Part model, mm, in its own coordinate system. Give positions to 0.01 mm unless a question says otherwise; leave off trailing zeros. Loops run counter-clockwise (first coordinate to the right, second up) from the corner with the lowest first, then second, coordinate; pieces in that order, holes last. Notation, with made-up numbers: M 23.5,77 L 28.5,77 A24 ccw 28.5,91 Z; hole C 54,2.25 d2. An arc over 180 degrees is marked long. Answer in a Markdown table with one row per item.
Autodesk Inventor part; units mm, degrees
ref_plane "YZ Plane" through (0, 0, 0) normal (1, 0, 0) x (0, 1, 0)
ref_plane "XZ Plane" through (0, 0, 0) normal (0, 1, 0) x (-1, 0, 0)
ref_plane "XY Plane" through (0, 0, 0) normal (0, 0, 1) x (1, 0, 0)
sketch "Sketch1" plane through (0, 0, 0) normal (0, 1, 0) x (-1, 0, 0)
  line L0 (38.1, 76.2) -> (-38.1, 76.2)
  line L1 (-38.1, 76.2) -> (-38.1, -76.2)
  line L2 (-38.1, -76.2) -> (38.1, -76.2)
  line L3 (38.1, -76.2) -> (38.1, 76.2)
  line L4 (38.1, 76.2) -> (-38.1, -76.2) construction
  line L5 (-38.1, 76.2) -> (38.1, -76.2) construction
  point P0 (0, 0)
  dimension "d0" = 76.2
  dimension "d1" = 152.4
extrude "Extrusion1" add sketch "Sketch1" along normal blind 6.35
sketch "Sketch2" plane through (0, 6.35, 0) normal (0, 1, 0) x (1, 0, 0)
  line L0 (38.1, 76.2) -> (-38.1, 76.2)
  line L1 (-38.1, 76.2) -> (-38.1, -76.2)
  line L2 (38.1, -76.2) -> (38.1, 76.2)
  line L3 (-38.1, -76.2) -> (38.1, -76.2)
  point P0 (0, 0)
  point P1 (-25.4, 63.5)
  point P2 (25.4, 63.5)
  point P3 (25.4, -63.5)
  point P4 (-25.4, -63.5)
  dimension "d11" = 12.7
  dimension "d12" = 12.7
  dimension "d13" = 12.7
  dimension "d14" = 12.7
  dimension "d15" = 12.7
  dimension "d16" = 12.7
  dimension "d17" = 12.7
  dimension "d18" = 12.7
hole "Hole1" at (-25.4, 6.35, -63.5) at (25.4, 6.35, -63.5) at (25.4, 6.35, 63.5) at (-25.4, 6.35, 63.5) direction (0, -1, 0) diameter 6.7564 depth 10.8 tip angle 118
sketch "Sketch3" plane through (0, 6.35, 0) normal (0, 1, 0) x (1, 0, 0)
  line L0 (-38.1, -76.2) -> (38.1, -76.2)
  line L1 (-38.1, 76.2) -> (-38.1, -76.2)
  line L2 (38.1, -76.2) -> (38.1, 76.2)
  line L3 (38.1, 76.2) -> (-38.1, 76.2)
  point P0 (0, 0)
  point P1 (-25.4, 44.45)
  point P2 (-25.4, -44.45)
  point P3 (25.4, -44.45)
  point P4 (25.4, 46.482)
  dimension "d26" = 31.75
  dimension "d27" = 12.7
  dimension "d28" = 31.75
  dimension "d29" = 12.7
  dimension "d30" = 12.7
  dimension "d32" = 31.75
  dimension "d33" = 12.7
  dimension "d34" = 90.932
hole "Hole2" at (-25.4, 6.35, -44.45) at (-25.4, 6.35, 44.45) at (25.4, 6.35, 44.45) at (25.4, 6.35, -46.482) direction (0, -1, 0) diameter 2.6416 depth 10.9728 tip angle 118
properties part number "GalvoBoardPlate"
(1) Pin check, flat tip, straight feed: pin 1 Ø5.5 at (x, z) = (25.4, -63.5) entering from +Y. Stop position of the tip, or through.
Recorded:
| item | result |
|---|---|
| pin 1 | passes through |
(2) Pull direction X, two halves, no side cores. Call faces 1 (the face through (38.1, 3, 1)), 2 (the face through (25.003, 3.131, -45.222)), 3 (the face through (1, 3, -76.2)): +X half, -X half, draft (parallel to the pull), parting line (faces both ways), or undercut.
Recorded:
| item | result |
|---|---|
| face 1 | +X half |
| face 2 | undercut |
| face 3 | draft |
(3) Drill centre lines: line 1 along X through (y, z) = (3.5, 63.5); line 2 along Z through (x, y) = (-25.4, 4.75); line 3 along Z through (x, y) = (25.4, 2). Where is each one in solid material? Low to high.
Recorded:
| item | result |
|---|---|
| line 1 | x = -38.1 to -28.78, -22.02 to 22.02, 28.78 to 38.1 |
| line 2 | z = -76.2 to -66.88, -60.12 to -45.77, -43.13 to 43.13, 45.77 to 60.12, 66.88 to 76.2 |
| line 3 | z = -76.2 to -66.88, -60.12 to -47.8, -45.16 to 43.13, 45.77 to 60.12, 66.88 to 76.2 |
(4) Saw through at A-A (z = -63.5). Write the cut outline in (x, y).
Recorded:
| item | result |
|---|---|
| outline | M -38.1,0 L -28.78,0 L -28.78,6.35 L -38.1,6.35 Z; M -22.02,0 L 22.02,0 L 22.02,6.35 L -22.02,6.35 Z; M 28.78,0 L 38.1,0 L 38.1,6.35 L 28.78,6.35 Z |
